Solid Edge part; units mm, degrees
sketch "Sketch1" plane through (0, 0, 0) normal (0, 0, 1) x (1, 0, 0)
  circle A0 centre (-35.7272, 13.2376) radius 2
extrude "Protrusion1" add sketch "Sketch1" along normal blind 5.7
sketch "Sketch2" plane through (-35.7272, 13.2376, 5.7) normal (0, 0, 1) x (1, 0, 0)
  circle A0 centre (0, 0) radius 4
extrude "kopdia8" add sketch "Sketch2" along normal blind 2.3
chamfer "kegel" distance 2 angle 45 1 edges at (-39.7272, 13.2376, 5.7)
cosmetic_thread "Thread1"
sketch "Sketch3" plane through (-35.7272, 13.2376, 8) normal (0, 0, 1) x (1, 0, 0)
  line L0 (-0.7217, 1.25) -> (0.7217, 1.25)
  line L1 (0.7217, 1.25) -> (1.4434, 0)
  line L2 (1.4434, 0) -> (0.7217, -1.25)
  line L3 (0.7217, -1.25) -> (-0.7217, -1.25)
  line L4 (-0.7217, -1.25) -> (-1.4434, 0)
  line L5 (-1.4434, 0) -> (-0.7217, 1.25)
extrude "zeskant" cut sketch "Sketch3" against normal blind 2
Model file for the job. Use its own axes, mm. A direction names the side the tool comes from. Give positions to 0.01 mm unless a question says otherwise; leave off trailing zeros. Order: outer loops, then holes, each group sorted by start corner. A loop starts at its lowest first (then second) coordinate and runs counter-clockwise, first axis right, second up. Notation, with made-up numbers: (45.25, -3.75) - (57.25, -3.75) arc R37 cw to (57.25, 32.25) - close; hole circle Ø2 at (-16.5, 61.25). An arc over 180 degrees is marked (long way). One line per item, written item: value.
Item 1: Two-plate mould, pull along X, no slides. Class faces 4 (the cylindrical face through (-31.91, 12.04, 7.85)), 5 (the flat face through (-34.64, 12.62, 7.01)), 6 (the flat face through (-36, 13, 0)): released by +X, released by -X, zero draft, split by the parting line, or undercut.
Response values:
face 4: split by the parting line
face 5: undercut
face 6: zero draft
Item 2: Slice it at A-A (z = 6.75). List the corners of the cut face in (x, y), then the cut area to 3 significant figures.
Response values:
outline: circle Ø6.1 at (-35.73, 13.24); hole (-37.17, 13.24) - (-36.45, 11.99) - (-35.01, 11.99) - (-34.28, 13.24) - (-35.01, 14.49) - (-36.45, 14.49) - close
area: 23.8 mm2
Item 3: Wall check: line 1 (X direction, y = 12.5, z = 6.5); line 2 (Z direction, x = -36, y = 14.25); line 3 (X direction, y = 15, z = 6). Give the ranges that are in metal, low to high.
Response values:
line 1: -38.43 to -36.74, -34.71 to -33.03
line 2: 0 to 6
line 3: -37.21 to -34.25
Item 4: Pin check, flat tips, straight feed: pin 1 Ø0.7 at (x, z) = (-35.5, 7) entering from -Y; pin 2 Ø1.5 at (x, z) = (-33, 6.5) entering from +Y; pin 3 Ø1.5 at (x, y) = (-38.5, 15.5) entering from -Z. Stop position of each tip, or through.
Response values:
pin 1: y = 9.59
pin 2: y = 15.76
pin 3: z = 6.53
Item 5: Slice it at B-B (z = 1.5). List the corners of the cut face in (x, y), then the cut area to 3 significant figures.
Response values:
outline: circle Ø4 at (-35.73, 13.24)
area: 12.6 mm2
Item 6: Tool access for faces 1 (the flat face through (-37, 14, 8)), 2 (the flat face through (-36, 13, 6)), 3 (the cylindrical face through (-33.88, 14, 2.81)): list every direction of +Z, -Z, +X, -X, +Y, -Y with a clear straight run to the whole face (end or side of a thin tool).
Response values:
face 1: +Z, +X, -X, +Y, -Y
face 2: +Z
face 3: -Z
